Design review of the part built by this model. Coordinates are the model's own, in mm. Face numbers are marked on the shaded views. A direction names the side the tool comes from. Give positions to 0.01 mm unless a question says otherwise; leave off trailing zeros. Write each loop counter-clockwise with the first axis right and the second up, starting at its lowest first coordinate (ties: lowest second). Pieces come first, ordered by that corner, then holes. Notation, with made-up numbers: M 12,-3.75 L 49,-3.75 A20 cw 49,7.25 Z; hole C 4.5,-35 d4. An arc over 180 degrees is marked long. Write each question's results on one line, items separated by ' | '. Start each with the question number.
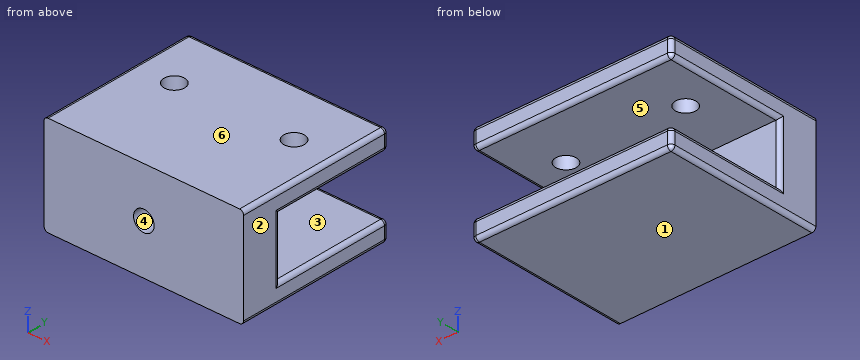
from build123d import *

# Parameters (mm, degrees)
SKETCH1_W           = 50
SKETCH1_H           = 25
BOSS_EXTRUDE1_DEPTH = 40
SKETCH2_W           = 50
SKETCH2_H           = 15
CUT_EXTRUDE1_DEPTH  = 30
FILLET1_R           = 1
CUT_EXTRUDE2_REACH  = 55.385
SKETCH3_R           = 2.5796875
SKETCH3_R_2         = 2.579687
SKETCH4_R           = 2.57968
CUT_EXTRUDE3_DEPTH  = 8


with BuildPart() as part:
    # Sketch1 → Boss-Extrude1 (new body)
    with BuildSketch(Plane(origin=(0, 0, 0), x_dir=(1, 0, 0), z_dir=(0, 1, 0))):
        Rectangle(SKETCH1_W, SKETCH1_H)
    extrude(amount=BOSS_EXTRUDE1_DEPTH)

    # Sketch2 → Cut-Extrude1 (cut)
    with BuildSketch(Plane(origin=(0, 40, 0), x_dir=(1, 0, 0), z_dir=(0, 1, 0))):
        Rectangle(SKETCH2_W, SKETCH2_H)
    extrude(amount=-CUT_EXTRUDE1_DEPTH, mode=Mode.SUBTRACT)

    # Fillet1
    fillet1_edges = [part.edges().sort_by_distance(p)[0] for p in [
        (-25, 40, -10),
        (0, 40, 12.5),
        (25, 40, -10),
        (-25, 40, 10),
        (25, 10, 0),
        (25, 25, -7.5),
        (25, 25, 7.5),
        (-25, 10, 0),
        (-25, 25, 7.5),
        (-25, 25, -7.5),
        (0, 40, -7.5),
        (0, 40, 7.5),
        (25, 40, 10),
        (0, 40, -12.5),
        (25, 20, 12.5),
        (-25, 20, 12.5),
        (-25, 20, -12.5),
        (25, 20, -12.5),
    ]]
    fillet(fillet1_edges, radius=FILLET1_R)

    # Sketch3 → Cut-Extrude2 (cut, up to next)
    with BuildSketch(Plane.XY.offset(12.5), mode=Mode.PRIVATE) as cut_extrude2_sk1:
        with Locations((-15, 25)):
            Circle(SKETCH3_R)
    cut_extrude2_tool1 = extrude(cut_extrude2_sk1.sketch, amount=-CUT_EXTRUDE2_REACH, mode=Mode.PRIVATE) & part.part
    # Sketch3 → Cut-Extrude2 (cut, up to next)
    with BuildSketch(Plane.XY.offset(12.5), mode=Mode.PRIVATE) as cut_extrude2_sk2:
        with Locations((15, 25)):
            Circle(SKETCH3_R_2)
    cut_extrude2_tool2 = extrude(cut_extrude2_sk2.sketch, amount=-CUT_EXTRUDE2_REACH, mode=Mode.PRIVATE) & part.part
    add(cut_extrude2_tool1.solids().sort_by_distance((-15, 25, 12.5))[0], mode=Mode.SUBTRACT)
    add(cut_extrude2_tool2.solids().sort_by_distance((15, 25, 12.5))[0], mode=Mode.SUBTRACT)

    # Sketch4 → Cut-Extrude3 (cut)
    with BuildSketch(Plane(origin=(0, 0, 0), x_dir=(-1, 0, 0), z_dir=(0, -1, 0))):
        with Locations(Location((0, 0, 0), (0, 0, 90))):
            Circle(SKETCH4_R)
    extrude(amount=-CUT_EXTRUDE3_DEPTH, mode=Mode.SUBTRACT)


solid = part.part
Q1. Wall thickness on line 1 along X through (y, z) = (6, 0); line 2 along Z through (x, y) = (10, 19); line 3 along Y through (x, z) = (-15, 9.05): over which ranges is each line inside the solid? List them lowest first. Write a range as from..to.
Q2. The part is to be moulded in two halves that separate along Z. For the marked faces 1, 2 and 3, say which applies: pulls with the +Z half, pulls with the -Z half, needs draft (parallel to the pull), parting line crosses it, or undercut.
Q3. We need section C-C on y = 25. Write out the cut boundary in (x, z), and give its area (3 significant figures).
Q4. For pin 1 Ø5 at (x, z) = (19, -1.5) entering from +Y; pin 2 Ø4.5 at (x, z) = (0, 0) entering from -Y, all flat-tipped, find the tip position at first contact; note any pin that passes through.
Q5. We need section A-A on y = 14. Write out the cut boundary in (x, z).
Q6. We need section B-B on z = 9.5. Write out the cut boundary in (x, y), and give its area (3 significant figures).
Q7. We need section D-D on x = -14. Write out the cut boundary in (y, z).
Q8. For the marked faces 4, 5 and 6, list the 3-axis set-ups (+Z, -Z, +X, -X, +Y, -Y) from which the entire face can be reached by the end or side of a thin tool; tool diameter is ignored.
Answer sheet:
1) line 1: -25..-2.58, 2.58..25 | line 2: -12.5..-7.5, 7.5..12.5 | line 3: 0..22.42, 27.58..40
2) face 1: pulls with the -Z half | face 2: needs draft | face 3: undercut
3) outline: M -25,-11.5 A1 ccw -24,-12.5 L 24,-12.5 A1 ccw 25,-11.5 L 25,-8.5 A1 ccw 24,-7.5 L -24,-7.5 A1 ccw -25,-8.5 Z; M -25,8.5 A1 ccw -24,7.5 L -17.58,7.5 L -17.58,12.5 L -24,12.5 A1 ccw -25,11.5 Z; M -12.42,7.5 L 12.42,7.5 L 12.42,12.5 L -12.42,12.5 Z; M 17.58,7.5 L 24,7.5 A1 ccw 25,8.5 L 25,11.5 A1 ccw 24,12.5 L 17.58,12.5 Z | area: 447 mm^2
4) pin 1: y = 10 | pin 2: y = 8
5) outline: M -25,-11.5 A1 ccw -24,-12.5 L 24,-12.5 A1 ccw 25,-11.5 L 25,-8.5 A1 ccw 24,-7.5 L -24,-7.5 A1 ccw -25,-8.5 Z; M -25,8.5 A1 ccw -24,7.5 L 24,7.5 A1 ccw 25,8.5 L 25,11.5 A1 ccw 24,12.5 L -24,12.5 A1 ccw -25,11.5 Z
6) outline: M -25,0 L 25,0 L 25,39 A1 ccw 24,40 L -24,40 A1 ccw -25,39 Z; hole C -15,25 d5.16; hole C 15,25 d5.16 | area: 1,960 mm^2
7) outline: M 0,-12.5 L 39,-12.5 A1 ccw 40,-11.5 L 40,-8.5 A1 ccw 39,-7.5 L 10,-7.5 L 10,7.5 L 22.62,7.5 L 22.62,12.5 L 0,12.5 Z; M 27.38,7.5 L 39,7.5 A1 ccw 40,8.5 L 40,11.5 A1 ccw 39,12.5 L 27.38,12.5 Z
8) face 4: -Y | face 5: +X, -X, +Y | face 6: +Z, +X, -X, +Y, -Y
